Can you work these out from the drawing? Everything is in mm from the part's minimum corner. A direction names the side the tool comes from. Give positions to 0.01 mm unless a question says otherwise; leave off trailing zeros. Order: outer loops, then holes, each group sorted by start corner. A loop starts at its lowest first (then second) coordinate and runs counter-clockwise, first axis right, second up. Notation, with made-up numbers: M -37,-6 L -2,-6 A26 cw -2,24 Z; hole C 69,78 d3. An arc over 180 degrees is marked long. Answer in a Markdown table with one row per item. Add a question column.
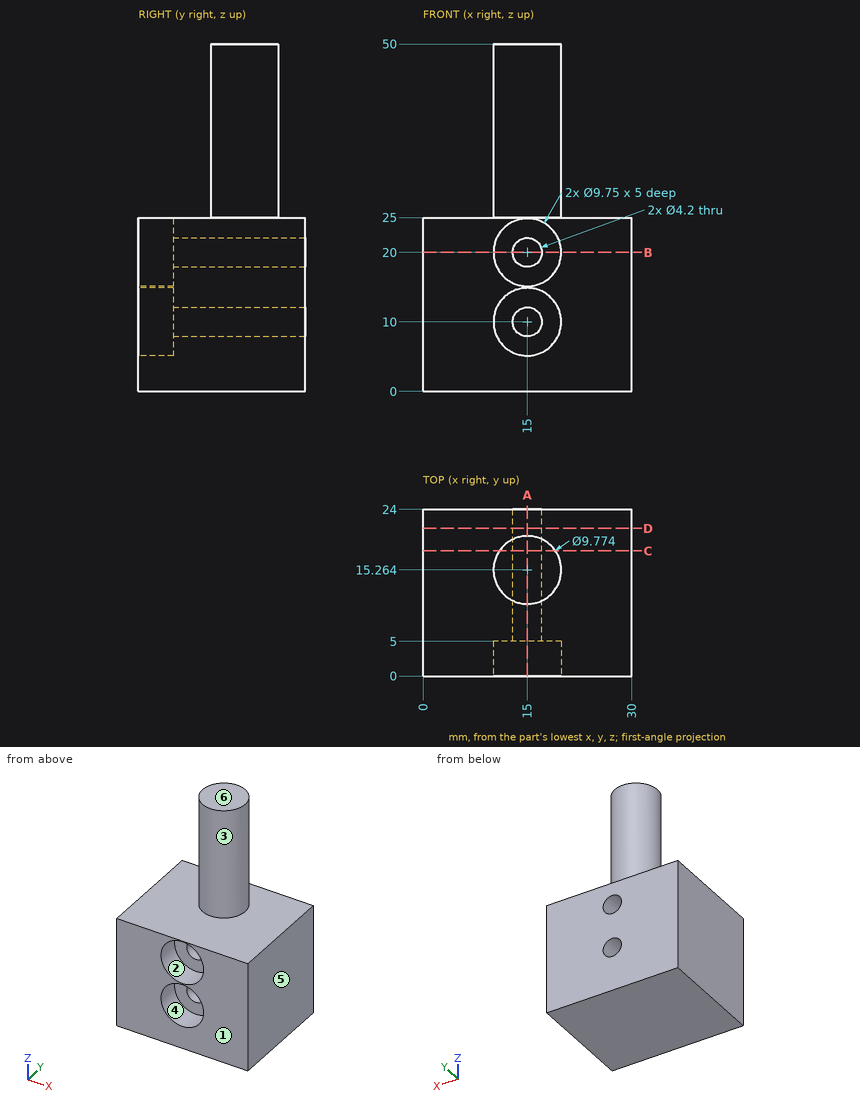
1. If I drill on line 1 along Z through (x, y) = (15, 9); line 2 along Z through (x, y) = (24.5, 5); line 3 along Y through (x, z) = (15, 28), over which ranges is the centre line in solid material (lowest first)? Write a range as [from, to].
2. Suppose I cut it at B-B on z = 20. List the corners of the cut face in (x, y) for me (1 decimal).
3. Suppose I cut it at C-C on y = 18. List the corners of the cut face in (x, z) for me, plus the area to 3 significant figures.
4. For the marked faces 1, 2 and 3, which set-ups out of +Z, -Z, +X, -X, +Y, -Y let a thin tool reach every point of the face, with its end or its side?
5. Thinking about a two-plate mould opening in Z: for the marked faces 4, 5 and 6, which applies, pulls with the +Z half, pulls with the -Z half, needs draft (parallel to the pull), parting line crosses it, or undercut?
6. Suppose I cut it at D-D on y = 21.25. List the corners of the cut face in (x, z) for me, plus the area to 3 significant figures.
7. Suppose I cut it at A-A on x = 15. Count the separate pieces of the cut face and the enclosed holes in it, plus the area to 3 significant figures.
8. Will these pins go through, and if not, where does the flat tip stop? P1, Ø1.5, axis at x = 4, y = 14.5, coming from the +Z side; P2, Ø5, axis at x = 13, z = 10.5, coming from the -Y side.
Findings below:
| question | item | result |
|---|---|---|
| 1 | line 1 | [0, 7.9], [12.1, 17.9], [22.1, 25] |
| 1 | line 2 | [0, 25] |
| 1 | line 3 | [10.38, 20.15] |
| 2 | outline | M 0,0 L 10.1,0 L 10.1,5 L 12.9,5 L 12.9,24 L 0,24 Z; M 17.1,5 L 19.9,5 L 19.9,0 L 30,0 L 30,24 L 17.1,24 Z |
| 3 | outline | M 0,0 L 30,0 L 30,25 L 19.05,25 L 19.05,50 L 10.95,50 L 10.95,25 L 0,25 Z; hole C 15,10 d4.2; hole C 15,20 d4.2 |
| 3 | area | 925 mm2 |
| 4 | face 1 | +Z, -Z, +X, -X, -Y |
| 4 | face 2 | -Y |
| 4 | face 3 | +Z |
| 5 | face 4 | undercut |
| 5 | face 5 | needs draft |
| 5 | face 6 | pulls with the +Z half |
| 6 | outline | M 0,0 L 30,0 L 30,25 L 0,25 Z; hole C 15,10 d4.2; hole C 15,20 d4.2 |
| 6 | area | 722 mm2 |
| 7 | separate pieces | 3 |
| 7 | enclosed holes | 0 |
| 7 | area | 587 mm2 |
| 8 | P1 | z = 25 |
| 8 | P2 | y = 5 |
